```python
from build123d import *

# Parameters (mm, degrees)
F0_W     = 165.1
F0_H     = 38.1
F1_DEPTH = 50.8
F2_W     = 76.2
F2_H     = 69.85
F3_DEPTH = 31.75
F5_W     = 6.35
F5_H     = 50.8
F6_DEPTH = 30.1625
F7_W     = 69.85
F7_H     = 57.15
F8_DEPTH = 3.175
F9_R     = 19.05
F10_R    = 19.05
F11_R    = 19.05


with BuildPart() as f1:
    # F0 (on Front) → F1 (new body, symmetric)
    with BuildSketch(Plane.XZ):
        with Locations((-22.901768, -7.525502)):
            Rectangle(F0_W, F0_H)
    extrude(amount=F1_DEPTH, both=True)

    # F2 (on face) → F3 (cut)
    with BuildSketch(Plane.XY.offset(11.524498)):
        with Locations((-61.001768, 3.175)):
            Rectangle(F2_W, F2_H)
    extrude(amount=-F3_DEPTH, mode=Mode.SUBTRACT)

    # F5 (on face) → F6 (cut)
    with BuildSketch(Plane.XY.offset(11.524498)):
        with Locations((-102.276768, -6.35)):
            Rectangle(F5_W, F5_H)
    extrude(amount=-F6_DEPTH, mode=Mode.SUBTRACT)

    # F7 (on face) → F8 (cut)
    with BuildSketch(Plane.XY.offset(11.524498)):
        with Locations((12.023232, -3.175)):
            Rectangle(F7_W, F7_H)
    extrude(amount=-F8_DEPTH, mode=Mode.SUBTRACT)

    # F9
    f9_edges = [f1.edges().sort_by_distance(p)[0] for p in [
        (-105.451768, -50.8, -7.525502),
    ]]
    fillet(f9_edges, radius=F9_R)

    # F10
    f10_edges = [f1.edges().sort_by_distance(p)[0] for p in [
        (59.648232, -50.8, -7.525502),
    ]]
    fillet(f10_edges, radius=F10_R)

    # F11
    f11_edges = [f1.edges().sort_by_distance(p)[0] for p in [
        (59.648232, 50.8, -7.525502),
        (-105.451768, 50.8, -7.525502),
    ]]
    fillet(f11_edges, radius=F11_R)


solid = f1.part
```
Design review of the part built by this model. Coordinates are the model's own, in mm. A direction names the side the tool comes from. Give positions to 0.01 mm unless a question says otherwise; leave off trailing zeros. Order: outer loops, then holes, each group sorted by start corner. A loop starts at its lowest first (then second) coordinate and runs counter-clockwise, first axis right, second up. Notation, with made-up numbers: M -31,65.5 L 9,65.5 A25 cw 9,89.5 Z; hole C 38.5,41.5 d2. An arc over 180 degrees is marked long. One line per question, with ' | ' between items. Start each with the question number.
Q1. We need section C-C (z = -6). Write out the cut boundary in (x, y), plus the area to 3 significant figures.
Q2. For pin 1 Ø7 at (x, y) = (-103.5, -5.5) entering from +Z; pin 2 Ø3.5 at (y, z) = (3.5, 10.5) entering from -X; pin 3 Ø1.5 at (y, z) = (-10, -18) entering from -X; pin 4 Ø5 at (x, y) = (-57.5, -27) entering from +Z, all flat-tipped, find the tip position at first contact; note any pin that passes through.
Q3. We need section D-D (x = 30). Write out the cut boundary in (y, z).
Q4. The part is to be moulded in two halves that separate along X. For faces 4 (the face through (-100.02, -45.07, -7.26)), 5 (the face through (-24, 50.8, -7)), 6 (the face through (-62, 38.1, -4)), say which applies: +X half, -X half, draft (parallel to the pull), parting line (faces both ways), or undercut.
Q5. Machinability: for faces 1 (the face through (-62, 4, -20.226)), 2 (the face through (-105.452, 14, -20)), 3 (the face through (-102, -6, -18.638)), which of the approach directions +Z, -Z, +X, -X, +Y, -Y give a long, thin tool a straight path to every point of the face, cutting with its end or side? Answer none if there is none.
Q6. We need section A-A (y = -19). Write out the cut boundary in (x, z).
Q7. For L1, parallel to Y at x = -56, z = -20; L2, parallel to X at y = -17, z = -19, list the stretches that pass through material, from the lowest coordinate up. Write a range as [from, to].
Q8. We need section B-B (x = -26). Write out the cut boundary in (y, z).
Returned:
1) outline: M -105.45,-31.75 A19.05 ccw -86.4,-50.8 L 40.6,-50.8 A19.05 ccw 59.65,-31.75 L 59.65,31.75 A19.05 ccw 40.6,50.8 L -86.4,50.8 A19.05 ccw -105.45,31.75 L -105.45,19.05 L -99.1,19.05 L -99.1,38.1 L -22.9,38.1 L -22.9,-31.75 Z | area: 10,800 mm2
2) pin 1: z = -18.64 | pin 2: x = 46.95 | pin 3: x = -105.45 | pin 4: z = -20.23
3) outline: M -50.8,-26.58 L 50.8,-26.58 L 50.8,11.52 L 25.4,11.52 L 25.4,8.35 L -31.75,8.35 L -31.75,11.52 L -50.8,11.52 Z
4) face 4: -X half | face 5: draft | face 6: undercut
5) face 1: +Z | face 2: +Z, -Z, -X, +Y, -Y | face 3: +Z, -X
6) outline: M -105.45,-26.58 L 59.65,-26.58 L 59.65,11.52 L 46.95,11.52 L 46.95,8.35 L -22.9,8.35 L -22.9,-20.23 L -99.1,-20.23 L -99.1,-18.64 L -105.45,-18.64 Z
7) L1: [-50.8, -31.75], [38.1, 50.8] | L2: [-105.45, -99.1], [-22.9, 59.65]
8) outline: M -50.8,-26.58 L 50.8,-26.58 L 50.8,11.52 L 38.1,11.52 L 38.1,-20.23 L -31.75,-20.23 L -31.75,11.52 L -50.8,11.52 Z
